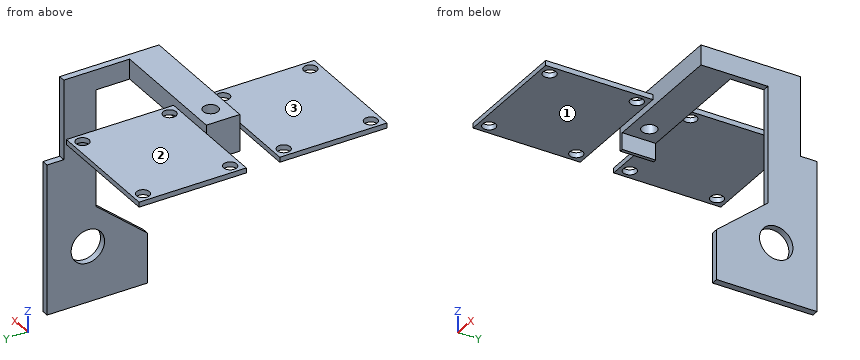
Autodesk Inventor part; units mm, degrees
ref_plane "YZ Plane" through (0, 0, 0) normal (1, 0, 0) x (0, 1, 0)
ref_plane "XZ Plane" through (0, 0, 0) normal (0, 1, 0) x (-1, 0, 0)
ref_plane "XY Plane" through (0, 0, 0) normal (0, 0, 1) x (1, 0, 0)
sketch "Sketch14" plane through (0, 0, 0) normal (0, 0, 1) x (1, 0, 0)
  line L0 (0, 0) -> (-6.08, 0)
  line L1 (-6.08, 0) -> (0, 0)
  line L2 (0, 0) -> (6.08, 0)
  line L3 (-6.08, 0) -> (-6.08, 5)
  line L4 (-6.08, 0) -> (-1.08, 0) construction
  line L5 (-6.08, 5) -> (6.08, 5)
  line L6 (6.08, 5) -> (6.08, -5)
  line L7 (6.08, -5) -> (-6.08, -5)
  line L8 (-6.08, -5) -> (-6.08, 5)
  dimension "d66" = 6.08
  dimension "d67" = 6.08
  dimension "d68" = 5
  dimension "d69" = 90
  dimension "d70" = 12.16
  dimension "d71" = 10
extrude "Extrusion7" add sketch "Sketch14" along normal blind 2
sketch "Sketch15" plane through (0, 0, 2) normal (0, 0, 1) x (1, 0, 0)
  circle A0 centre (0, 0) radius 1.0665
hole "Hole4" at (0, 0, 2) direction (0, 0, -1) diameter 4.5 end through all
sketch "Sketch16" plane through (0, 0, 2) normal (0, 0, 1) x (1, 0, 0)
  line L0 (6.08, 5) -> (-6.08, 5)
  line L1 (0, 5) -> (10, 5)
  line L2 (10, 5) -> (-25.7, 5)
  line L3 (-25.7, 5) -> (-25.7, 37.05)
  line L4 (-25.7, 37.05) -> (10, 37.05)
  line L5 (10, 37.05) -> (10, 5)
  line L6 (-6.08, -5) -> (6.08, -5)
  line L7 (0, -5) -> (10, -5)
  line L8 (10, -5) -> (-25.7, -5)
  line L9 (-25.7, -5) -> (-25.7, -37.05)
  line L10 (-25.7, -37.05) -> (10, -37.05)
  line L11 (10, -37.05) -> (10, -5)
  line L12 (-25.7, 37.05) -> (-22.7, 37.05)
  line L13 (-22.7, 37.05) -> (-22.7, 34.05)
  line L14 (-22.7, 34.05) -> (-25.7, 34.05)
  line L15 (-25.7, 34.05) -> (-25.7, 37.05)
  line L16 (-22.7, 34.05) -> (7, 34.05)
  line L17 (7, 34.05) -> (7, 8)
  line L18 (7, 8) -> (-22.7, 8)
  line L19 (-22.7, 8) -> (-22.7, 34.05)
  line L20 (-25.7, -37.05) -> (-22.7, -37.05)
  line L21 (-22.7, -37.05) -> (-22.7, -34.05)
  line L22 (-22.7, -34.05) -> (-25.7, -34.05)
  line L23 (-25.7, -34.05) -> (-25.7, -37.05)
  line L24 (-22.7, -34.05) -> (7, -34.05)
  line L25 (7, -34.05) -> (7, -8)
  line L26 (7, -8) -> (-22.7, -8)
  line L27 (-22.7, -8) -> (-22.7, -34.05)
  line L28 (-25.7, -5) -> (10, -5)
  line L29 (10, -5) -> (10, -37.05)
  line L30 (10, -37.05) -> (-25.7, -37.05)
  line L31 (-25.7, -37.05) -> (-25.7, -5)
  point P0 (0, 0)
  dimension "d81" = 10
  dimension "d82" = 35.7
  dimension "d83" = 32.05
  dimension "d84" = 35.7
  dimension "d85" = 32.05
  dimension "d86" = 3
  dimension "d87" = 3
  dimension "d88" = 29.7
  dimension "d89" = 26.05
  dimension "d90" = 3
  dimension "d91" = 3
  dimension "d92" = 29.7
  dimension "d93" = 26.05
  dimension "d172" = 10
extrude "Extrusion8" add sketch "Sketch16" along normal blind 1.5 contours L16 L17 L18 L19 | L0 L2 L3 L14 L13 L4 L5 L1 | L13 L14 L3 L4 | L27 L26 L25 L24 | L6 L7 L11 L10 L21 L22 L9 L8 | L22 L21 L10 L9
hole "Hole5" at (-22.7, 34.05, 2) at (-22.7, 8, 2) at (7, 8, 2) at (7, 34.05, 2) at (7, -8, 2) at (7, -34.05, 2) at (-22.7, -34.05, 2) at (-22.7, -8, 2) direction (0, 0, 1) diameter 3.9 end through all
sketch "Sketch17" plane through (0, 0, 2) normal (0, 0, 1) x (1, 0, 0)
  circle A0 centre (0, 0) radius 2.25
  line L0 (6.08, -5) -> (6.08, 5)
  line L1 (6.08, 5) -> (-6.08, 5)
  line L2 (-6.08, 5) -> (-6.08, -5)
  line L3 (-6.08, -5) -> (6.08, -5)
extrude "Extrusion9" add sketch "Sketch17" along normal blind 4
sketch "Sketch18" plane through (6.08, -5, 0) normal (1, 0, 0) x (0, 0, -1)
  line L0 (0, 0) -> (0, 10)
  line L1 (0, 10) -> (-2, 10)
  line L2 (-3.5, 10) -> (-2, 10)
  line L3 (-3.5, 10) -> (-6, 10)
  line L4 (-6, 0) -> (-6, 10)
  line L5 (-3.5, 0) -> (-6, 0)
  line L6 (-2, 0) -> (-3.5, 0)
  line L7 (0, 0) -> (-2, 0)
  point P0 (0, 5)
extrude "Extrusion10" add sketch "Sketch18" along normal blind 35
sketch "Sketch19" plane through (41.08, -5, 0) normal (1, 0, 0) x (0, 0, -1)
  line L0 (-6, 10) -> (-6, 0)
  line L1 (-6, 0) -> (-16, 0)
  line L2 (-16, 0) -> (-16, 50)
  line L3 (-16, 50) -> (29, 50)
  line L4 (29, 50) -> (29, 25)
  line L5 (29, 25) -> (0, 10)
  line L6 (0, 10) -> (0, 0)
  line L7 (0, 10) -> (0, 0)
  line L8 (0, 0) -> (-6, 0)
  point P0 (0, 5)
  dimension "d107" = 10
  dimension "d108" = 50
  dimension "d109" = 90
  dimension "d110" = 45
  dimension "d111" = 90
  dimension "d112" = 25
extrude "Extrusion11" add sketch "Sketch19" along normal blind 2.5
sketch "Sketch21" plane through (43.58, -5, 0) normal (1, 0, 0) x (0, 0, -1)
  line L0 (-3.5, 10) -> (-6, 10)
  line L1 (0, 10) -> (0, 24.05)
  line L2 (0, 10) -> (14.05, 10) construction
  line L3 (0, 24.05) -> (6.713, 24.05)
  point P0 (0, 5)
  point P1 (3, 10)
  point P2 (-2, 10)
  dimension "d118" = 14.05
  dimension "d119" = 90
  dimension "d120" = 6.713
  dimension "d121" = 90
hole "Hole6" at (43.58, 19.05, -6.713) direction (-1, 0, 0) diameter 10 end through all
sketch "Sketch22" plane through (43.58, -5, 0) normal (1, 0, 0) x (0, 0, -1)
  circle A0 centre (6.713, 24.05) radius 5
  line L0 (6.713, 24.05) -> (6.713, 32.05)
  line L1 (6.713, 24.05) -> (14.713, 24.05) construction
  line L2 (6.713, 32.05) -> (24.213, 32.05)
  line L3 (24.213, 32.05) -> (-10.787, 32.05)
  point P0 (0, 5)
  dimension "d129" = 8
  dimension "d130" = 90
  dimension "d131" = 17.5
  dimension "d132" = 90
  dimension "d133" = 35
hole "Hole7" at (43.58, 27.05, 10.787) at (43.58, 27.05, -24.213) direction (-1, 0, 0) diameter 4.2 end through all
sketch "Sketch23" plane through (43.58, -5, 0) normal (1, 0, 0) x (0, 0, -1)
  line L0 (-3.5, 0) -> (-2, 0)
  line L1 (-2, 0) -> (-2, -9)
  line L2 (-2, 0) -> (7, 0) construction
  line L3 (-2, -9) -> (33, -9) construction
  line L4 (-2, -9) -> (33, -9)
  line L5 (-2, -9) -> (33, -9) construction
  line L6 (33, -9) -> (40.7782, -1.2218)
  line L7 (40.7782, -1.2218) -> (60.7782, -1.2218)
  line L8 (33, -9) -> (68, -9)
  line L9 (33, -9) -> (68, -9) construction
  line L10 (68, -9) -> (68, -1.2218)
  line L11 (68, -1.2218) -> (60.7782, -1.2218)
  line L12 (68, -9) -> (68, -29)
  line L13 (68, -9) -> (88, -9) construction
  line L14 (68, -29) -> (-2, -29)
  line L15 (-2, -29) -> (-2, -9)
  line L16 (33, -9) -> (44.45, -9)
  line L17 (44.45, -9) -> (44.45, -13.669)
  line L18 (44.45, -9) -> (49.119, -9) construction
  line L19 (44.45, -13.669) -> (44.45, -21.669)
  line L20 (44.45, -21.669) -> (61.95, -21.669)
  line L21 (61.95, -21.669) -> (26.95, -21.669)
  circle A0 centre (26.95, -21.669) radius 2.1
  circle A1 centre (61.95, -21.669) radius 2.1
  circle A2 centre (44.45, -13.669) radius 5
  point P0 (0, 5)
  dimension "d141" = 9
  dimension "d142" = 90
  dimension "d145" = 35
  dimension "d146" = 0
  dimension "d147" = 11
  dimension "d148" = 135
  dimension "d149" = 20
  dimension "d150" = 35
  dimension "d151" = 0
  dimension "d152" = 20
  dimension "d153" = 90
  dimension "d154" = 90
  dimension "d155" = 11.45
  dimension "d156" = 4.669
  dimension "d157" = 90
  dimension "d158" = 8
  dimension "d159" = 17.5
  dimension "d160" = 35
  dimension "d161" = 4.2
  dimension "d162" = 4.2
  dimension "d163" = 10
extrude "Extrusion13" add sketch "Sketch23" against normal blind 2 contours L4 L8 A2 L12 L14 L15 | L6 L7 L11 L10 L8 A2
sketch "Sketch24" plane through (43.58, -5, 0) normal (1, 0, 0) x (0, 0, -1)
  line L0 (-16, 50) -> (-16, 0)
  line L1 (-16, 0) -> (-16, -29)
  line L2 (68, -29) -> (-2, -29)
  line L3 (-16, -29) -> (-2, -29)
  line L4 (0, 0) -> (-2, 0)
  line L5 (-2, -29) -> (-2, 0)
  line L6 (-16, 0) -> (0, 0)
  line L7 (-2, 0) -> (-16, 0)
  point P0 (0, 5)
  point P1 (3, 0)
extrude "Extrusion14" add sketch "Sketch24" against normal blind 2
sketch "Sketch25" plane through (41.58, -5, 0) normal (-1, 0, 0) x (0, 0, 1)
  line L0 (2, -9) -> (-33, -9)
  line L1 (-33, -9) -> (2, -9)
  line L2 (2, -9) -> (2, -11)
  line L3 (2, -11) -> (-33, -11)
  line L4 (-33, -11) -> (-33, -9)
  line L5 (2, -11) -> (6, -11)
  line L6 (6, -11) -> (6, 0)
  line L7 (6, 0) -> (2, 0)
  line L8 (2, 0) -> (2, -11)
  point P0 (0, 5)
  point P1 (2, -9)
  dimension "d168" = 35
  dimension "d169" = 2
extrude "Extrusion15" add sketch "Sketch25" along normal blind 10
sketch "Sketch27" plane through (43.58, -5, 0) normal (1, 0, 0) x (0, 0, -1)
  line L0 (68, -29) -> (-16, -29)
  line L1 (-16, -29) -> (69.4034, -29)
  line L2 (69.4034, -29) -> (69.4034, 52.4533)
  line L3 (69.4034, 52.4533) -> (-16, 52.4533)
  line L4 (-16, 52.4533) -> (-16, -29)
  point P0 (0, 5)
extrude "Extrusion17" cut sketch "Sketch27" against normal up to surface (12 mm away)
sketch "Sketch28" plane through (0, 0, 0) normal (0, 0, -1) x (-1, 0, 0)
  line L0 (6.08, -5) -> (-10, -5)
  line L1 (6.08, 5) -> (-10, 5)
  line L2 (6.08, -5) -> (5.08, -5)
  line L3 (5.08, -5) -> (5.08, 5)
  line L4 (5.08, 5) -> (6.08, 5)
  line L5 (6.08, 5) -> (6.08, -5)
  point P0 (0, 0)
  dimension "d177" = 1
extrude "Extrusion18" add sketch "Sketch28" along normal blind 5
sketch "Sketch29" plane through (31.58, -5, 6) normal (1, 0, 0) x (0, 0, -1)
  line L0 (6, 10) -> (6, 20)
  line L1 (6, 20) -> (41, 20)
  line L2 (6, 20) -> (41, 20) construction
  line L3 (41, 20) -> (53.8558, 4.6791)
  line L4 (53.8558, 4.6791) -> (68.8558, 4.6791)
  line L5 (68.8558, 4.6791) -> (68.8558, 34.6791)
  line L6 (68.8558, 34.6791) -> (23.8558, 34.6791)
  line L7 (68.8558, 34.6791) -> (113.8558, 34.6791) construction
  line L8 (23.8558, 34.6791) -> (23.8558, 29.6791)
  line L9 (0, 10) -> (0, 0)
  line L10 (0, 10) -> (0, 29.6791)
  line L11 (0, 29.6791) -> (23.8558, 29.6791)
  line L12 (6, 10) -> (6, 0)
  line L13 (6, 0) -> (0, 0)
  line L14 (0, 0) -> (0, 10)
  point P0 (6, 5)
  dimension "d180" = 10
  dimension "d181" = 35
  dimension "d182" = 0
  dimension "d183" = 20
  dimension "d184" = 130
  dimension "d185" = 15
  dimension "d186" = 30
  dimension "d187" = 45
  dimension "d188" = 180
  dimension "d189" = 5
  dimension "d190" = 90
extrude "Extrusion19" add sketch "Sketch29" along normal blind 2
sketch "Sketch30" plane through (33.58, -5, 6) normal (1, 0, 0) x (0, 0, -1)
  line L0 (68.8558, 4.6791) -> (68.8558, 34.6791)
  line L1 (68.8558, 34.6791) -> (52.1638, 34.6791)
  line L2 (68.8558, 34.6791) -> (23.8558, 34.6791)
  line L3 (52.1638, 34.6791) -> (52.1638, 22.4901)
  circle A0 centre (52.1638, 22.4901) radius 5
  point P0 (6, 5)
  dimension "d193" = 16.692
  dimension "d194" = 12.189
  dimension "d195" = 10
extrude "Extrusion20" cut sketch "Sketch30" against normal blind 10
properties part number "Shelf_half"
Here's how the part is built. I have some questions about the finished solid (model axes, mm). Face numbers are marked on the shaded views. A direction names the side the tool comes from. Coordinates: 2 decimals unless noted, no trailing zeros. Order: outer loops, then holes, each group sorted by start corner. A loop starts at its lowest first (then second) coordinate and runs counter-clockwise, first axis right, second up.
1) Imagine slicing it at C-C on z = -42.5. List the corners of the cut face in (x, y) for me, and give its area (3 significant figures).
2) I need wall thicknesses on line 1 (X direction, y = 8, z = 2.6); line 2 (Y direction, x = 7, z = 3); line 3 (X direction, y = -34.05, z = 2.6). Which ranges of each line are inside material? Lowest first, please.
3) Imagine slicing it at B-B on x = 7. List the corners of the cut face in (y, z) for me.
4) Imagine slicing it at A-A on y = 34.05. List the corners of the cut face in (x, z) for me, and give its area (4 significant figures).
5) Will these pins go through, and if not, where does the flat tip stop? pin 1 (2 mm diameter, centred on y = 6.5, z = -54, fed in from -X); pin 2 (4.5 mm diameter, centred on x = 7, y = 8, fed in from -Z); pin 3 (1 mm diameter, centred on x = 32.5, z = -25.5, fed in from -Y).
6) Imagine slicing it at D-D on x = -15. List the corners of the cut face in (y, z) for me, and give its area (4 significant figures).
7) Which directions (+Z, -Z, +X, -X, +Y, -Y) give clear straight access to the entire face, cutting with the end or side of a thin tool? Please do the marked faces 1, 2 and 3.
Response values:
1. outline: (31.58, 6.06) - (33.58, 6.06) - (33.58, 14.09) - (31.58, 14.09) - close; (31.58, 20.89) - (33.58, 20.89) - (33.58, 29.68) - (31.58, 29.68) - close
1. area: 33.6 mm2
2. line 1: x = -25.7 to -24.65, -20.75 to 5.05, 8.95 to 10, 31.58 to 33.58
2. line 2: y = -37.05 to -36, -32.1 to -9.95, -6.05 to 6.05, 9.95 to 32.1, 36 to 37.05
2. line 3: x = -25.7 to -24.65, -20.75 to 5.05, 8.95 to 10
3. outline: (-37.05, 2) - (-36, 2) - (-36, 3.5) - (-37.05, 3.5) - close; (-32.1, 2) - (-9.95, 2) - (-9.95, 3.5) - (-32.1, 3.5) - close; (-6.05, 2) - (-5, 2) - (-5, 0) - (5, 0) - (5, 2) - (6.05, 2) - (6.05, 3.5) - (5, 3.5) - (5, 6) - (-5, 6) - (-5, 3.5) - (-6.05, 3.5) - close; (9.95, 2) - (32.1, 2) - (32.1, 3.5) - (9.95, 3.5) - close; (36, 2) - (37.05, 2) - (37.05, 3.5) - (36, 3.5) - close
4. outline: (-25.7, 2) - (-24.65, 2) - (-24.65, 3.5) - (-25.7, 3.5) - close; (-20.75, 2) - (5.05, 2) - (5.05, 3.5) - (-20.75, 3.5) - close; (8.95, 2) - (10, 2) - (10, 3.5) - (8.95, 3.5) - close
4. area: 41.85 mm2
5. pin 1: stops at x = 31.58
5. pin 2: stops at z = 2
5. pin 3: stops at y = 15
6. outline: (-37.05, 2) - (-5, 2) - (-5, 3.5) - (-37.05, 3.5) - close; (5, 2) - (37.05, 2) - (37.05, 3.5) - (5, 3.5) - close
6. area: 96.15 mm2
7. face 1: -Z, +X, -X, -Y
7. face 2: +Z, -X, +Y
7. face 3: +Z, +X, -X, -Y
